Could you check a few things on this drawing? It's one solid part, dimensions in mm from its lowest x, y, z. A direction names the side the tool comes from. Coordinates: 2 decimals unless noted, no trailing zeros. Write each loop counter-clockwise with the first axis right and the second up, starting at its lowest first coordinate (ties: lowest second). Pieces come first, ordered by that corner, then holes. Notation, with made-up numbers: (-16, 14.25) - (15, 14.25) arc R30 cw to (15, 39.25) - close; hole circle Ø2 at (-17, -2). An arc over 180 degrees is marked (long way). Use one line per item in the form item = value. Start each with the question number.
(1) If I drill on probe 1 along Z at (x, y) = (58.5, 25.5); probe 2 along X at (y, z) = (14, 4.75); probe 3 along Y at (x, z) = (44, 20.5) (1 decimal), over which ranges is the centre line in solid material (lowest first)? Write a range as from..to.
(2) On a 3-axis mill with a long thin cutter (end or side, diameter ignored), from which of +Z, -Z, +X, -X, +Y, -Y can I reach the whole of each face in a straight line? I mean the marked faces 1 and 2. Say none if no direction works.
(3) If we section it at D-D on y = 33.5: Please give me the cut outline in (x, z).
(4) If we section it at B-B on y = 22: Please give me the cut outline in (x, z), then the cut area to 3 significant figures.
(5) If we section it at A-A on x = 43.5: Please give me the cut outline in (y, z) (1 decimal).
(6) For pin 1 Ø5 at (x, y) = (37, 28) entering from +Z; pin 2 Ø6.5 at (x, z) = (28.5, 16) entering from -Y; pin 3 Ø10 at (x, z) = (49.5, 21.5) entering from +Y (1 decimal), each with a flat end and sliding along its axis, tell me the tip position at first contact or that it passes through.
(7) Thinking about a two-plate mould opening in X: for the marked faces 3, 4 and 5, which applies, pulls with the +X half, pulls with the -X half, needs draft (parallel to the pull), parting line crosses it, or undercut?
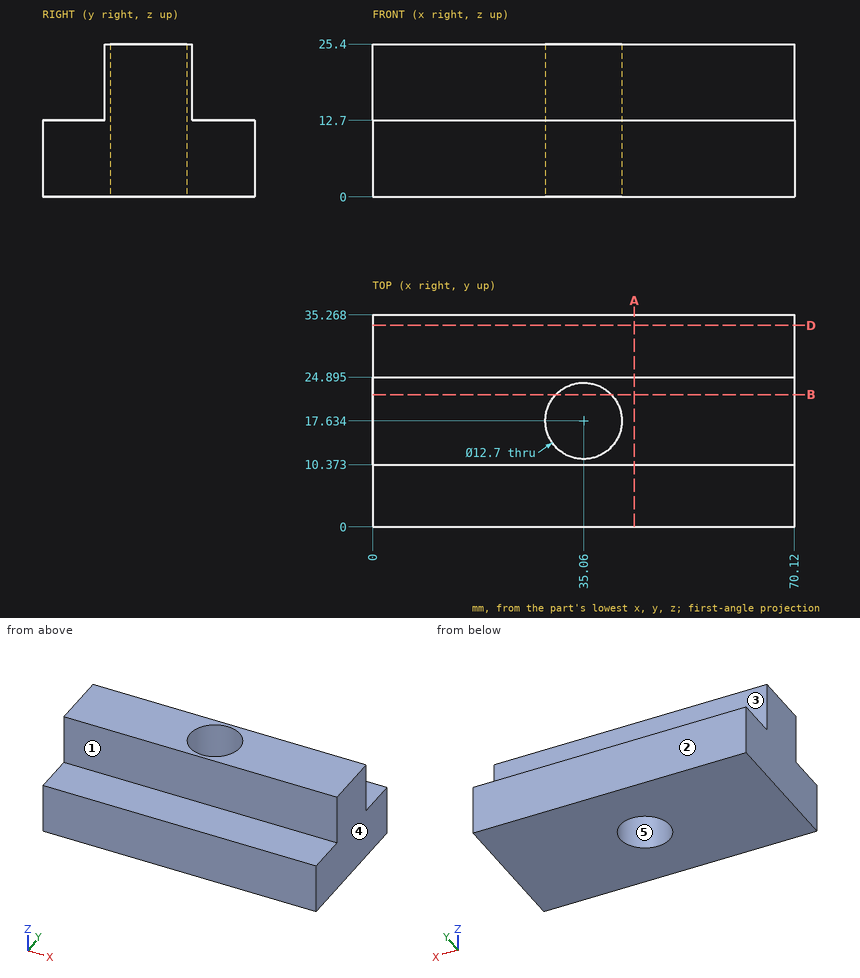
Reported:
q1.probe_1 = 0..12.7
q1.probe_2 = 0..29.85, 40.27..70.12
q1.probe_3 = 10.4..24.9
q2.face_1 = +Z, +X, -X, -Y
q2.face_2 = +Z, -Z, +X, -X, +Y
q3.outline = (0, 0) - (70.12, 0) - (70.12, 12.7) - (0, 12.7) - close
q4.outline = (0, 0) - (30.45, 0) - (30.45, 25.4) - (0, 25.4) - close; (39.67, 0) - (70.12, 0) - (70.12, 25.4) - (39.67, 25.4) - close
q4.area = 1,550 mm2
q5.outline = (0, 0) - (35.3, 0) - (35.3, 12.7) - (24.9, 12.7) - (24.9, 25.4) - (10.4, 25.4) - (10.4, 12.7) - (0, 12.7) - close
q6.pin_1 = 12.7
q6.pin_2 = 10.37
q6.pin_3 = 24.9
q7.face_3 = needs draft
q7.face_4 = pulls with the +X half
q7.face_5 = undercut
